Source: CAD feature listing. Evaluate the final solid. Frame: model axes, mm. A direction names the side the tool comes from. Round coordinates to 2 decimals unless told otherwise and drop trailing zeros. Loops run counter-clockwise (first coordinate to the right, second up) from the corner with the lowest first, then second, coordinate; pieces in that order, holes last.
Item 1: Ray query, L1, parallel to Y at x = 7.5, z = -33; L2, parallel to Y at x = 7.5, z = -15.5; L3, parallel to Z at x = -7.5, y = -1.5. Return the intervals inside material, ascending.
Item 2: First-contact query: P1, Ø5.5, axis at x = -9, z = -11, coming from the -Y side; P2, Ø3, axis at x = 8.75, z = -10.5, coming from the -Y side; P3, Ø6, axis at x = -8.75, z = -10.5, coming from the +Y side (3 decimals); P4, Ø4, axis at y = 19, z = -34, coming from the +X side. Flat tips, straight axial feed; report the tip coordinate or a pass-through.
Item 3: Section query A-A on z = -42. Return loops of the section in (x, y) (3 decimals).
Item 4: Pull-direction query (Y, two-part tool) for faces 5 (the cylindrical face through (0, 35, 1)), 6 (the cylindrical face through (6.3, -2.5, -10)), 7 (the cylindrical face through (9, 10, -23)); classes: released by +Y, released by -Y, zero draft, split by the parting line, or undercut.
Item 5: Section query C-C on z = -35.5. Give the number of separate pieces and of enclosed holes in the cut face, then the cut area to 3 significant figures.
Item 6: Section query B-B on y = 17.5. Return loops of the section in (x, z), then the cut area to 3 significant figures.
Item 7: Access query for faces 1 (the flat face through (-9, 0, -10)), 2 (the flat face through (0, 23, 0)), 3 (the flat face through (-10, 25.645, -23)), 4 (the cylindrical face through (-1.08, 12.62, 0.99)). Directions: +Z, -Z, +X, -X, +Y, -Y. A direction counts if a zero-diameter tool reaches every point of the face in a straight line with its end or side. Return the directions, or none.
Item 8: Section query D-D on y = 29. Return loops of the section in (x, z), then the cut area to 3 significant figures.
```python
from build123d import *

# Parameters (mm, degrees)
SKETCH1_R           = 5
SKETCH1_R_2         = 2
BOSS_EXTRUDE1_DEPTH = 2
SKETCH2_R           = 2
SKETCH2_R_2         = 5
BOSS_EXTRUDE2_DEPTH = 2
SKETCH4_R           = 3
SKETCH4_R_2         = 2.5
BOSS_EXTRUDE4_DEPTH = 46
BOSS_EXTRUDE5_REACH = 63.929
SKETCH8_R           = 5
SKETCH8_R_2         = 2.5
BOSS_EXTRUDE6_DEPTH = 5


with BuildPart() as part:
    # Sketch1 → Boss-Extrude1 (new body)
    with BuildSketch(Plane.XY):
        with BuildLine():
            Line((-17.5, 0), (17.5, 0))
            Line((17.5, 0), (11.704867869, 25.645008161))
            ThreePointArc((11.704867869, 25.645008161), (0, 35), (-11.704867869, 25.645008161))
            Line((-11.704867869, 25.645008161), (-17.5, 0))
        make_face()
        with Locations((0, 17.5)):
            Circle(SKETCH1_R, mode=Mode.SUBTRACT)
        with Locations((7.5, 8)):
            Circle(SKETCH1_R_2, mode=Mode.SUBTRACT)
        with Locations((-7.5, 8)):
            Circle(SKETCH1_R_2, mode=Mode.SUBTRACT)
        with Locations((0, 28)):
            Circle(SKETCH1_R_2, mode=Mode.SUBTRACT)
    extrude(amount=BOSS_EXTRUDE1_DEPTH)



with BuildPart() as body_2:
    # Sketch2 → Boss-Extrude2 (new body)
    with BuildSketch(Plane.XY.offset(-48)):
        with BuildLine():
            Line((17.5, 0), (11.704867869, 25.645008161))
            ThreePointArc((11.704867869, 25.645008161), (0, 35), (-11.704867869, 25.645008161))
            Line((-11.704867869, 25.645008161), (-17.5, 0))
            Line((-17.5, 0), (17.5, 0))
        make_face()
        with Locations((-7.5, 8)):
            Circle(SKETCH2_R, mode=Mode.SUBTRACT)
        with Locations((7.5, 8)):
            Circle(SKETCH2_R, mode=Mode.SUBTRACT)
        with Locations((0, 17.5)):
            Circle(SKETCH2_R_2, mode=Mode.SUBTRACT)
        with Locations((0, 28)):
            Circle(SKETCH2_R, mode=Mode.SUBTRACT)
    extrude(amount=BOSS_EXTRUDE2_DEPTH)


with BuildPart() as part_1:
    add(part.part)

    add(body_2.part)  # Boss-Extrude4 merges body 2
    # Sketch4 → Boss-Extrude4 (add)
    # profile 1 of 3: a face of its own
    with BuildSketch(Plane(origin=(0, 0, 0), x_dir=(-1, 0, 0), z_dir=(0, 0, -1))):
        with Locations(Location((7.5, 8, 0), (0, 0, 180))):
            Circle(SKETCH4_R)
        with Locations(Location((7.5, 8, 0), (0, 0, 180))):
            Circle(SKETCH4_R_2, mode=Mode.SUBTRACT)
    # profile 2 of 3: a face of its own
    with BuildSketch(Plane(origin=(0, 0, 0), x_dir=(-1, 0, 0), z_dir=(0, 0, -1))):
        with Locations(Location((0, 28, 0), (0, 0, 180))):
            Circle(SKETCH4_R)
        with Locations(Location((0, 28, 0), (0, 0, 180))):
            Circle(SKETCH4_R_2, mode=Mode.SUBTRACT)
    # profile 3 of 3: a face of its own
    with BuildSketch(Plane(origin=(0, 0, 0), x_dir=(-1, 0, 0), z_dir=(0, 0, -1))):
        with Locations(Location((-7.5, 8, 0), (0, 0, 180))):
            Circle(SKETCH4_R)
        with Locations(Location((-7.5, 8, 0), (0, 0, 180))):
            Circle(SKETCH4_R_2, mode=Mode.SUBTRACT)
    extrude(amount=BOSS_EXTRUDE4_DEPTH)

    # Sketch3 → Boss-Extrude5 (add, up to next)
    with BuildSketch(Plane(origin=(0, 0, 0), x_dir=(-1, 0, 0), z_dir=(0, 0, -1)), mode=Mode.PRIVATE) as boss_extrude5_sk1:
        Polygon((12.495241869, 4), (16.59609978, 4), (11.704867869, 25.645008161), (7.604009958, 25.645008161), align=None)
    boss_extrude5_tool1 = extrude(boss_extrude5_sk1.sketch, amount=BOSS_EXTRUDE5_REACH, mode=Mode.PRIVATE) - part_1.part
    # Sketch3 → Boss-Extrude5 (add, up to next)
    with BuildSketch(Plane(origin=(0, 0, 0), x_dir=(-1, 0, 0), z_dir=(0, 0, -1)), mode=Mode.PRIVATE) as boss_extrude5_sk2:
        Polygon((-16.59609978, 4), (-12.495241869, 4), (-7.604009958, 25.645008161), (-11.704867869, 25.645008161), align=None)
    boss_extrude5_tool2 = extrude(boss_extrude5_sk2.sketch, amount=BOSS_EXTRUDE5_REACH, mode=Mode.PRIVATE) - part_1.part
    # Sketch3 → Boss-Extrude5 (add, up to next)
    with BuildSketch(Plane(origin=(0, 0, 0), x_dir=(-1, 0, 0), z_dir=(0, 0, -1)), mode=Mode.PRIVATE) as boss_extrude5_sk3:
        Polygon((17.5, 0), (16.59609978, 4), (12.495241869, 4), (-12.495241869, 4), (-16.59609978, 4), (-17.5, 0), align=None)
    boss_extrude5_tool3 = extrude(boss_extrude5_sk3.sketch, amount=BOSS_EXTRUDE5_REACH, mode=Mode.PRIVATE) - part_1.part
    add(boss_extrude5_tool1.solids().sort_by_distance((-12.100055, 14.822504, 0))[0])
    add(boss_extrude5_tool2.solids().sort_by_distance((12.100055, 14.822504, 0))[0])
    add(boss_extrude5_tool3.solids().sort_by_distance((0, 1.982326, 0))[0])

    # Sketch8 → Boss-Extrude6 (add)
    # profile 1 of 4: a face of its own
    with BuildSketch(Plane.XZ):
        with Locations(Location((8.75, -10.5, 0), (0, 0, 90))):
            Circle(SKETCH8_R)
        with Locations(Location((8.75, -10.5, 0), (0, 0, 270))):
            Circle(SKETCH8_R_2, mode=Mode.SUBTRACT)
    # profile 2 of 4: a face of its own
    with BuildSketch(Plane.XZ):
        with Locations(Location((8.75, -35.5, 0), (0, 0, 90))):
            Circle(SKETCH8_R)
        with Locations(Location((8.75, -35.5, 0), (0, 0, 90))):
            Circle(SKETCH8_R_2, mode=Mode.SUBTRACT)
    # profile 3 of 4: a face of its own
    with BuildSketch(Plane.XZ):
        with Locations(Location((-8.75, -35.5, 0), (0, 0, 90))):
            Circle(SKETCH8_R)
        with Locations(Location((-8.75, -35.5, 0), (0, 0, 270))):
            Circle(SKETCH8_R_2, mode=Mode.SUBTRACT)
    # profile 4 of 4: a face of its own
    with BuildSketch(Plane.XZ):
        with Locations(Location((-8.75, -10.5, 0), (0, 0, 90))):
            Circle(SKETCH8_R)
        with Locations(Location((-8.75, -10.5, 0), (0, 0, 90))):
            Circle(SKETCH8_R_2, mode=Mode.SUBTRACT)
    extrude(amount=BOSS_EXTRUDE6_DEPTH)


solid = part_1.part
```
Data:
1. L1: y = -5 to 4, 5 to 5.5, 10.5 to 11
1. L2: y = 0 to 4, 5 to 5.5, 10.5 to 11
1. L3: z = -40.34 to -37.67, -33.33 to -30.66, -15.34 to -12.67, -8.33 to -5.66
2. P1: stops at y = -5
2. P2: stops at y = 0
2. P3: stops at y = 25.645
2. P4: stops at x = 13.66
3. outline: (-17.5, 0) - (17.5, 0) - (11.705, 25.645) - (7.604, 25.645) - (12.495, 4) - (-12.495, 4) - (-7.604, 25.645) - (-11.705, 25.645) - close; circle Ø6 at (-7.5, 8); circle Ø6 at (0, 28); circle Ø6 at (7.5, 8); hole circle Ø5 at (-7.5, 8); hole circle Ø5 at (0, 28); hole circle Ø5 at (7.5, 8)
4. face 5: released by +Y
4. face 6: zero draft
4. face 7: undercut
5. separate pieces: 4
5. enclosed holes: 3
5. area: 390 mm2
6. outline: (-13.55, -48) - (-5, -48) - (-5, -46) - (-9.44, -46) - (-9.44, 0) - (-5, 0) - (-5, 2) - (-13.55, 2) - close; (5, -48) - (13.55, -48) - (13.55, 2) - (5, 2) - (5, 0) - (9.44, 0) - (9.44, -46) - (5, -46) - close
6. area: 446 mm2
7. face 1: -Y
7. face 2: none
7. face 3: -X, +Y
7. face 4: +Z, -Z
8. outline: (-10.39, -48) - (-1.73, -48) - (-1.73, -46) - (-2.29, -46) - (-2.29, 0) - (-1.73, 0) - (-1.73, 2) - (-10.39, 2) - (-10.39, 0) - (-2.83, 0) - (-2.83, -46) - (-10.39, -46) - close; (1.73, -48) - (10.39, -48) - (10.39, -46) - (2.83, -46) - (2.83, 0) - (10.39, 0) - (10.39, 2) - (1.73, 2) - (1.73, 0) - (2.29, 0) - (2.29, -46) - (1.73, -46) - close
8. area: 119 mm2
